from build123d import *

# Parameters (mm, degrees)
SKETCH1_W           = 150
SKETCH1_H           = 15
BOSS_EXTRUDE1_DEPTH = 150
SKETCH2_W           = 75
SKETCH2_H           = 75
BOSS_EXTRUDE2_DEPTH = 150
SKETCH3_W           = 30
SKETCH3_H           = 30
BOSS_EXTRUDE3_DEPTH = 10
SKETCH4_W           = 75
SKETCH4_H           = 75
BOSS_EXTRUDE4_DEPTH = 150
LPATTERN1_COUNT     = 2
LPATTERN1_PITCH     = 160
SKETCH5_W           = 75
SKETCH5_H           = 75
BOSS_EXTRUDE5_DEPTH = 100


with BuildPart() as part:
    # Sketch1 → Boss-Extrude1 (new body)
    with BuildSketch(Plane.YZ):
        Rectangle(SKETCH1_W, SKETCH1_H)
    extrude(amount=BOSS_EXTRUDE1_DEPTH)

    # Sketch2 → Boss-Extrude2 (add)
    with BuildSketch(Plane.XY.offset(7.5)):
        with Locations((75, 0)):
            Rectangle(SKETCH2_W, SKETCH2_H)
    extrude(amount=BOSS_EXTRUDE2_DEPTH)

    # Sketch3 → Boss-Extrude3 (add)
    with BuildSketch(Plane.XY.offset(157.5)):
        with Locations((75, 0)):
            Rectangle(SKETCH3_W, SKETCH3_H)
    boss_extrude3 = extrude(amount=BOSS_EXTRUDE3_DEPTH)

    # Sketch4 → Boss-Extrude4 (add)
    with BuildSketch(Plane.XY.offset(167.5)):
        with Locations((75, 0)):
            Rectangle(SKETCH4_W, SKETCH4_H)
    extrude(amount=BOSS_EXTRUDE4_DEPTH)

    # LPattern1: Boss-Extrude3 ×2
    with Locations(*[(0, 0, i * LPATTERN1_PITCH) for i in range(1, LPATTERN1_COUNT)]):
        add(boss_extrude3)

    # Sketch5 → Boss-Extrude5 (add)
    with BuildSketch(Plane.XY.offset(327.5)):
        with Locations((75, 0)):
            Rectangle(SKETCH5_W, SKETCH5_H)
    extrude(amount=BOSS_EXTRUDE5_DEPTH)


solid = part.part
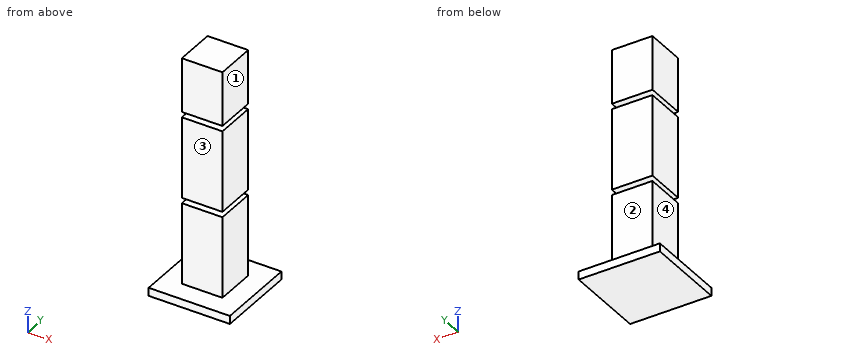
Design review of the part built by this model. Coordinates are the model's own, in mm. Face numbers are marked on the shaded views. A direction names the side the tool comes from. Give positions to 0.01 mm unless a question says otherwise; leave off trailing zeros. Order: outer loops, then holes, each group sorted by start corner. A loop starts at its lowest first (then second) coordinate and runs counter-clockwise, first axis right, second up. Notation, with made-up numbers: (-16, 67) - (17, 67) arc R16 ccw to (17, 96) - close; hole circle Ø1 at (57.25, 29). An arc over 180 degrees is marked (long way). Write item = value, one per line. Start each with the question number.
Q1. Tool access review of the marked faces 1, 2, 3 and 4: name each direction out of +Z, -Z, +X, -X, +Y, -Y from which nothing blocks a thin tool from reaching the whole face with its end or side.
Q2. We need section B-B on y = 27. State the section outline as (x, z) points.
Q3. We need section A-A on x = 53.5. State the section outline as (y, z) points, plus the area to 4 significant figures.
Q4. Clearance check with flat-ended pins moving along their axes: pin 1 Ø5 at (x, y) = (79, -50.5) entering from +Z; pin 2 Ø10 at (x, z) = (71.5, 180.5) entering from -Y; pin 3 Ø5 at (y, z) = (-5.5, 322) entering from -X. State where each tip first meets the part, or that it passes through.
Q5. We need section C-C on y = -1.5. State the section outline as (x, z) points, plus the area to 4 significant figures.
Q6. To check wall thickness, follow L1, parallel to Z at x = 93, y = 20.5; L2, parallel to Z at x = 11.5, y = 35; L3, parallel to Y at x = 106, z = 55. State the ranges of each line that lie inside material, in increasing order. Write a range as from..to.
Q7. We need section D-D on x = 16. State the section outline as (y, z) points, plus the area to 3 significant figures.
Working result:
q1.face_1 = +Z, +X, +Y, -Y
q1.face_2 = +Z, +X, -X, +Y
q1.face_3 = +Z, +X, -X, -Y
q1.face_4 = +Z, -X, +Y, -Y
q2.outline = (0, -7.5) - (150, -7.5) - (150, 7.5) - (112.5, 7.5) - (112.5, 157.5) - (37.5, 157.5) - (37.5, 7.5) - (0, 7.5) - close; (37.5, 167.5) - (112.5, 167.5) - (112.5, 317.5) - (37.5, 317.5) - close; (37.5, 327.5) - (112.5, 327.5) - (112.5, 427.5) - (37.5, 427.5) - close
q3.outline = (-75, -7.5) - (75, -7.5) - (75, 7.5) - (37.5, 7.5) - (37.5, 157.5) - (-37.5, 157.5) - (-37.5, 7.5) - (-75, 7.5) - close; (-37.5, 167.5) - (37.5, 167.5) - (37.5, 317.5) - (-37.5, 317.5) - close; (-37.5, 327.5) - (37.5, 327.5) - (37.5, 427.5) - (-37.5, 427.5) - close
q3.area = 32,250 mm²
q4.pin_1 = 7.5
q4.pin_2 = -37.5
q4.pin_3 = 60
q5.outline = (0, -7.5) - (150, -7.5) - (150, 7.5) - (112.5, 7.5) - (112.5, 157.5) - (90, 157.5) - (90, 167.5) - (112.5, 167.5) - (112.5, 317.5) - (90, 317.5) - (90, 327.5) - (112.5, 327.5) - (112.5, 427.5) - (37.5, 427.5) - (37.5, 327.5) - (60, 327.5) - (60, 317.5) - (37.5, 317.5) - (37.5, 167.5) - (60, 167.5) - (60, 157.5) - (37.5, 157.5) - (37.5, 7.5) - (0, 7.5) - close
q5.area = 32,850 mm²
q6.L1 = -7.5..157.5, 167.5..317.5, 327.5..427.5
q6.L2 = -7.5..7.5
q6.L3 = -37.5..37.5
q7.outline = (-75, -7.5) - (75, -7.5) - (75, 7.5) - (-75, 7.5) - close
q7.area = 2,250 mm²
